Print and shaded views of the part. All mm, measured from the part's lowest x, y and z. Coordinates: 2 decimals unless noted, no trailing zeros. Loops run counter-clockwise (first coordinate to the right, second up) from the corner with the lowest first, then second, coordinate; pieces in that order, holes last. Notation, with made-up numbers: M 10,77.25 L 58,77.25 A13 ccw 58,81.25 Z; hole C 63,57 d10. An arc over 180 degrees is marked long. Use a Markdown table: item, result. Add a question column.
1) Band-saw the part on A-A (x = 30). List the corners of the cut face in (y, z), plus the area to 4 significant figures.
2) Band-saw the part on D-D (x = 11). List the corners of the cut face in (y, z).
3) Wall check: probe 1 along Z at (x, y) = (11, 1.5); probe 2 along X at (y, z) = (6.5, 80); probe 3 along X at (y, z) = (3.25, 89). Give the ranges that are in metal, low to high. Write a range as from..to.
4) Pull direction Z, two halves, no side cores. Call the marked faces 1 and 2: released by +Z, released by -Z, zero draft, split by the parting line, or undercut.
5) Band-saw the part on B-B (z = 33). List the corners of the cut face in (x, y).
6) Pin check, flat tip, straight feed: pin 1 Ø14 at (x, z) = (30, 78) entering from -Y. Stop position of the tip, or through.
7) Band-saw the part on C-C (y = 1.25). List the corners of the cut face in (x, z), plus the area to 3 significant figures.
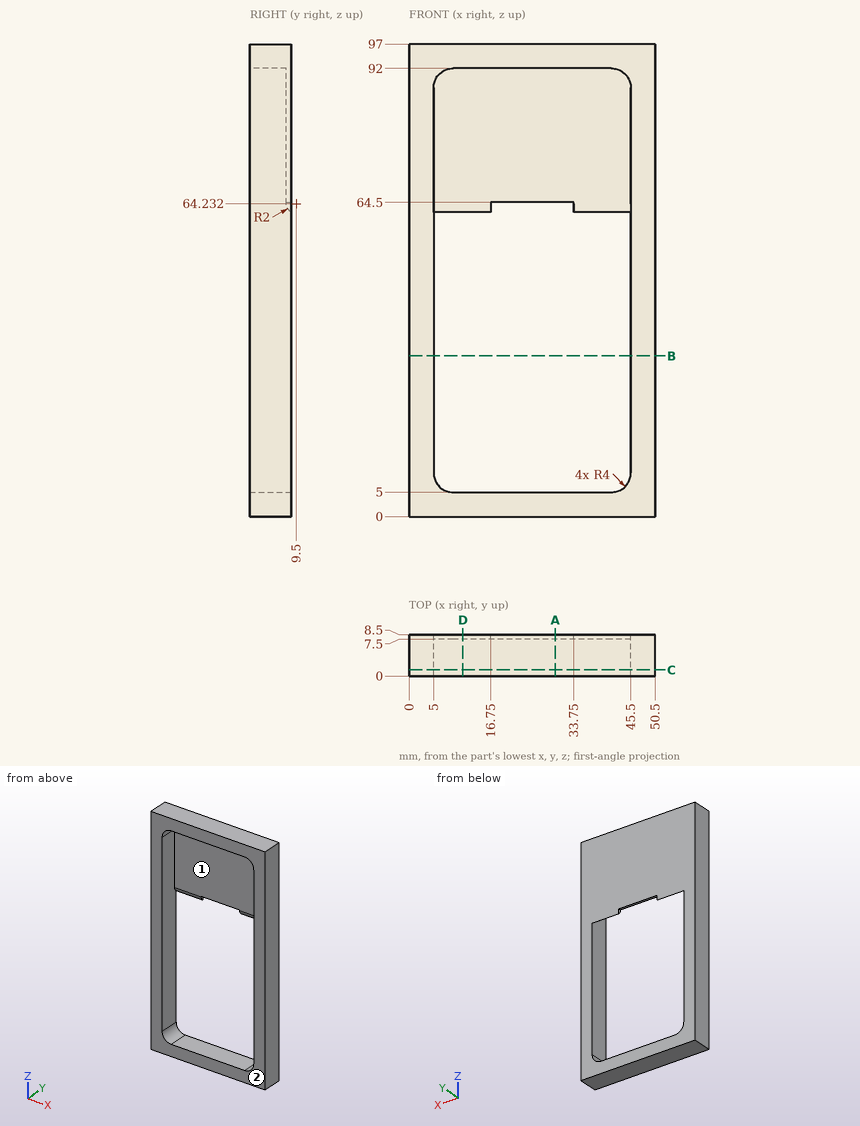
Entries:
| question | item | result |
|---|---|---|
| 1 | outline | M 0,0 L 8.5,0 L 8.5,5 L 0,5 Z; M 0,92 L 7.5,92 L 7.5,64.5 L 8.5,64.5 L 8.5,97 L 0,97 Z |
| 1 | area | 112.5 mm2 |
| 2 | outline | M 0,0 L 8.5,0 L 8.5,5 L 0,5 Z; M 0,92 L 7.5,92 L 7.5,64.23 A2 ccw 8.5,62.5 L 8.5,97 L 0,97 Z |
| 3 | probe 1 | 0..5, 92..97 |
| 3 | probe 2 | 0..5, 45.5..50.5 |
| 3 | probe 3 | 0..5.13, 45.37..50.5 |
| 4 | face 1 | undercut |
| 4 | face 2 | zero draft |
| 5 | outline | M 0,0 L 5,0 L 5,8.5 L 0,8.5 Z; M 45.5,0 L 50.5,0 L 50.5,8.5 L 45.5,8.5 Z |
| 6 | pin 1 | y = 7.5 |
| 7 | outline | M 0,0 L 50.5,0 L 50.5,97 L 0,97 Z; hole M 5,9 A4 ccw 9,5 L 41.5,5 A4 ccw 45.5,9 L 45.5,88 A4 ccw 41.5,92 L 9,92 A4 ccw 5,88 Z |
| 7 | area | 1,390 mm2 |
